Check sheet for the modelled part. Datum: model origin and axes. Units: mm. Round coordinates to 2 decimals unless told otherwise and drop trailing zeros. Write each loop counter-clockwise with the first axis right and the second up, starting at its lowest first coordinate (ties: lowest second). Pieces come first, ordered by that corner, then holes. Notation, with made-up numbers: (45, 71) -> (77, 71) arc R18 ccw to (77, 78) -> close; hole circle Ø1 at (15, 8.5). An arc over 180 degrees is marked (long way). One line per item, written item: value. Start each with the question number.
```python
from build123d import *

# Parameters (mm, degrees)
BOSS_EXTRUDE4_DEPTH = 200
CUT_EXTRUDE5_DEPTH  = 45
BOSS_EXTRUDE5_DEPTH = 7.5
BOSS_EXTRUDE6_DEPTH = 7.5


with BuildPart() as part:
    # Sketch1 → Boss-Extrude4 (new body)
    with BuildSketch(Plane.XY):
        with BuildLine():
            Line((22.5, 19.843134833), (154.787565553, -130.156865167))
            ThreePointArc((154.787565553, -130.156865167), (152.130700386, -172.5), (109.787565553, -169.843134833))
            Line((109.787565553, -169.843134833), (-22.5, -19.843134833))
            ThreePointArc((-22.5, -19.843134833), (-19.843134833, 22.5), (22.5, 19.843134833))
        make_face()
    extrude(amount=BOSS_EXTRUDE4_DEPTH)

    # Sketch4 → Cut-Extrude5 (cut)
    with BuildSketch(Plane(origin=(22.5, 19.843134833, 0), x_dir=(0, 0, -1), z_dir=(0.75, 0.661437828, 0))):
        with BuildLine():
            Line((-192.5, 51.321419616), (-192.5, -204.008189627))
            ThreePointArc((-192.5, -204.008189627), (-182.248737342, -228.756926968), (-157.5, -239.008189627))
            Line((-157.5, -239.008189627), (-42.5, -239.008189627))
            ThreePointArc((-42.5, -239.008189627), (-17.751262658, -228.756926968), (-7.5, -204.008189627))
            Line((-7.5, -204.008189627), (-7.5, 51.321419616))
            Line((-7.5, 51.321419616), (-192.5, 51.321419616))
        make_face()
    extrude(amount=-CUT_EXTRUDE5_DEPTH, mode=Mode.SUBTRACT)

    # Sketch5 → Boss-Extrude5 (add)
    with BuildSketch(Plane(origin=(0, 0, 0), x_dir=(-1, 0, 0), z_dir=(0, 0, -1))):
        with BuildLine():
            ThreePointArc((-22.5, 19.843134833), (6.347313412, 29.320839218), (28.692196557, 8.761156129))
            Line((28.692196557, 8.761156129), (13.012632005, 60.110674556))
            Line((13.012632005, 60.110674556), (-22.5, 19.843134833))
        make_face()
    extrude(amount=-BOSS_EXTRUDE5_DEPTH)

    # Sketch6 → Boss-Extrude6 (add)
    with BuildSketch(Plane(origin=(0, 0, 192.5), x_dir=(-1, 0, 0), z_dir=(0, 0, -1))):
        Polygon((-20.631911768, 21.961347785), (13.012632005, 60.110674556), (28.692196557, 8.761156129), align=None)
    extrude(amount=-BOSS_EXTRUDE6_DEPTH)


solid = part.part
```
1. Cross-section at C-C (y = -7). Record the cut outline in (x, z).
2. Cross-section at B-B (z = 166.5). Record the cut outline in (x, y), plus the area to 3 significant figures.
3. Release check for a two-part mould opening along Z. For faces 1 (the face through (44.57, -95.893, 98.6)), 2 (the face through (144.501, -159.754, 9.404)), 3 (the face through (59, -68, 0)), 4 (the face through (146.254, -161.741, 189.562)) record: +Z half, -Z half, draft (parallel to the pull), parting line (faces both ways), or undercut.
4. Depth check by flat-ended pin: pin 1 Ø2 at (x, z) = (64.5, 91) entering from -Y; pin 2 Ø3 at (y, z) = (-61.5, 103.5) entering from -X (3 decimals); pin 3 Ø2 at (x, z) = (-4.5, 26) entering from +Y. Enter the tip coordinate at first touch or a pass-through.
5. Material ranges on probe 1 along Z at (x, y) = (104, -137); probe 2 along X at (y, z) = (-119.5, 144); probe 3 along Y at (x, z) = (55, 46.5), recorded low to high.
6. Cross-section at A-A (x = 7). Record the cut outline in (y, z), plus the area to 3 significant figures.
Working result:
1. outline: (-29.17, 0) -> (46.17, 0) -> (46.17, 7.5) -> (-13.83, 7.5) -> (-13.83, 192.5) -> (46.17, 192.5) -> (46.17, 200) -> (-29.17, 200) -> close
2. outline: (-28.43, 9.56) arc R30 ccw to (-22.5, -19.84) -> (109.79, -169.84) arc R30 ccw to (138.22, -179.41) -> close
2. area: 3,550 mm^2
3. face 1: draft
3. face 2: undercut
3. face 3: -Z half
3. face 4: undercut
4. pin 1: stops at y = -119.63
4. pin 2: stops at x = 12.915
4. pin 3: stops at y = -16.44
5. probe 1: z = 0 to 7.5, 192.5 to 200
5. probe 2: x = 65.39 to 85.39
5. probe 3: y = -107.72 to -85.04
6. outline: (-53.29, 0) -> (37.42, 0) -> (37.42, 7.5) -> (-30.62, 7.5) -> (-30.62, 192.5) -> (37.42, 192.5) -> (37.42, 200) -> (-53.29, 200) -> close
6. area: 5,560 mm^2
